from build123d import *

# Parameters (mm, degrees)
SKETCH1_R           = 15
BOSS_EXTRUDE1_DEPTH = 1


with BuildPart() as part:
    # Sketch1 → Boss-Extrude1 (new body)
    with BuildSketch(Plane(origin=(0, 0, 0), x_dir=(1, 0, 0), z_dir=(0, 1, 0))):
        with BuildLine():
            Line((37.587704831, -13.680805733), (18.793852416, -6.840402867))
            ThreePointArc((18.793852416, -6.840402867), (14.142135624, -14.142135624), (6.840402867, -18.793852416))
            Line((6.840402867, -18.793852416), (13.680805733, -37.587704831))
            ThreePointArc((13.680805733, -37.587704831), (0, -40), (-13.680805733, -37.587704831))
            Line((-13.680805733, -37.587704831), (-6.840402867, -18.793852416))
            ThreePointArc((-6.840402867, -18.793852416), (-14.142135624, -14.142135624), (-18.793852416, -6.840402867))
            Line((-18.793852416, -6.840402867), (-37.587704831, -13.680805733))
            ThreePointArc((-37.587704831, -13.680805733), (-39.061857441, -8.612275732), (-39.855769231, -3.393767674))
            ThreePointArc((-39.855769231, -3.393767674), (-39.69750686, -2.763455807), (-39.185267857, -2.363516773))
            ThreePointArc((-39.185267857, -2.363516773), (-37.5, 0), (-39.185267857, 2.363516773))
            ThreePointArc((-39.185267857, 2.363516773), (-39.69750686, 2.763455807), (-39.855769231, 3.393767674))
            ThreePointArc((-39.855769231, 3.393767674), (-39.061857441, 8.612275732), (-37.587704831, 13.680805733))
            Line((-37.587704831, 13.680805733), (-18.793852416, 6.840402867))
            ThreePointArc((-18.793852416, 6.840402867), (-14.142135624, 14.142135624), (-6.840402867, 18.793852416))
            Line((-6.840402867, 18.793852416), (-13.680805733, 37.587704831))
            ThreePointArc((-13.680805733, 37.587704831), (0, 40), (13.680805733, 37.587704831))
            Line((13.680805733, 37.587704831), (6.840402867, 18.793852416))
            ThreePointArc((6.840402867, 18.793852416), (14.142135624, 14.142135624), (18.793852416, 6.840402867))
            Line((18.793852416, 6.840402867), (37.587704831, 13.680805733))
            ThreePointArc((37.587704831, 13.680805733), (40, 0), (37.587704831, -13.680805733))
        make_face()
        with Locations(Location((0, 0, 0), (0, 0, 270))):
            Circle(SKETCH1_R, mode=Mode.SUBTRACT)
    extrude(amount=BOSS_EXTRUDE1_DEPTH)


solid = part.part
Geometry: final body of the model. Coordinates: model frame, mm. A direction names the side the tool comes from. Round coordinates to 2 decimals unless told otherwise and drop trailing zeros. Order: outer loops, then holes, each group sorted by start corner. A loop starts at its lowest first (then second) coordinate and runs counter-clockwise, first axis right, second up. Notation, with made-up numbers: (34.5, 86.5) -> (45.5, 86.5) arc R10 cw to (45.5, 104.5) -> close; hole circle Ø11 at (30.5, -14). An arc over 180 degrees is marked (long way). Put each result on its own line as item: value. Start each with the question number.
Q1. Section B-B on y = 0.55. Return the cut outline in (x, z), and give its area (3 significant figures).
Q2. Section A-A on x = 0. Return the cut outline in (y, z).
Q3. Reachability of faces 4 (the flat face through (-28.059, 0.493, 10.213)), 5 (the flat face through (10.213, 0.493, 28.059)), 6 (the flat face through (-28.3, 0.5, -10.3)) from +Z, -Z, +X, -X, +Y, -Y: full face, straight path, thin tool, end or side. Return the list, or none.
Q4. Section D-D on x = -9. Return the cut outline in (y, z).
Q5. Line query: probe 1 along Z at (x, y) = (-18, 0.75); probe 2 along Z at (x, y) = (20.5, 0.7); probe 3 along X at (y, z) = (0.45, -27.5). Output: solid intervals per line, ascending.
Q6. Section C-C on z = 0. Return the cut outline in (x, y), and give its area (3 significant figures).
Q7. Pull-direction query (Z, two-part tool) for faces 1 (the cylindrical face through (40, 0.5, -0.2)), 2 (the flat face through (28.059, 0.493, -10.213)), 3 (the cylindrical face through (14.228, 0.493, 14.055)); classes: +Z half, -Z half, draft (parallel to the pull), parting line (faces both ways), or undercut.
Ans:
1. outline: (-39.86, -3.39) arc R40 ccw to (-37.59, -13.68) -> (-18.79, -6.84) arc R20 ccw to (-6.84, -18.79) -> (-13.68, -37.59) arc R40 ccw to (13.68, -37.59) -> (6.84, -18.79) arc R20 ccw to (18.79, -6.84) -> (37.59, -13.68) arc R40 ccw to (37.59, 13.68) -> (18.79, 6.84) arc R20 ccw to (6.84, 18.79) -> (13.68, 37.59) arc R40 ccw to (-13.68, 37.59) -> (-6.84, 18.79) arc R20 ccw to (-18.79, 6.84) -> (-37.59, 13.68) arc R40 ccw to (-39.86, 3.39) arc R1 ccw to (-39.19, 2.36) arc R2.5 cw to (-39.19, -2.36) arc R1 ccw to start; hole circle Ø30 at (0, 0)
1. area: 2,220 mm2
2. outline: (0, -40) -> (1, -40) -> (1, -15) -> (0, -15) -> close; (0, 15) -> (1, 15) -> (1, 40) -> (0, 40) -> close
3. face 4: +Z, +Y, -Y
3. face 5: +X, +Y, -Y
3. face 6: -Z, +Y, -Y
4. outline: (0, -38.97) -> (1, -38.97) -> (1, -24.73) -> (0, -24.73) -> close; (0, -17.86) -> (1, -17.86) -> (1, -12) -> (0, -12) -> close; (0, 12) -> (1, 12) -> (1, 17.86) -> (0, 17.86) -> close; (0, 24.73) -> (1, 24.73) -> (1, 38.97) -> (0, 38.97) -> close
5. probe 1: z = -8.72 to 8.72
5. probe 2: z = -7.46 to 7.46
5. probe 3: x = -10.01 to 10.01
6. outline: (-37.5, 0) -> (-15, 0) -> (-15, 1) -> (-37.5, 1) -> close; (15, 0) -> (40, 0) -> (40, 1) -> (15, 1) -> close
6. area: 47.5 mm2
7. face 1: parting line
7. face 2: -Z half
7. face 3: undercut
